```python
from build123d import *

# Parameters (mm, degrees)
SKETCH1_W           = 10
SKETCH1_H           = 10
SKETCH1_W_2         = 8
SKETCH1_H_2         = 8
BOSS_EXTRUDE1_DEPTH = 500
CUT_EXTRUDE1_REACH  = 502.125
SKETCH2_R           = 1.6
CUT_EXTRUDE2_REACH  = 502.125
SKETCH3_R           = 1.6
SKETCH4_R           = 1.6
CUT_EXTRUDE3_DEPTH  = 10
SKETCH5_R           = 3.25
CUT_EXTRUDE4_DEPTH  = 1


with BuildPart() as part:
    # Sketch1 → Boss-Extrude1 (new body)
    with BuildSketch(Plane.XY):
        Rectangle(SKETCH1_W, SKETCH1_H)
        Rectangle(SKETCH1_W_2, SKETCH1_H_2, mode=Mode.SUBTRACT)
    extrude(amount=BOSS_EXTRUDE1_DEPTH)

    # Cut-Extrude1: up to this face of the body (flat: up to its plane)
    cut_extrude1_end = Plane(part.part.faces().sort_by_distance((0, -5, 250))[0])
    # Sketch2 → Cut-Extrude1 (cut, up to the picked face)
    with BuildSketch(Plane(origin=(0, 5, 0), x_dir=(1, 0, 0), z_dir=(0, 1, 0)), mode=Mode.PRIVATE) as cut_extrude1_sk1:
        with Locations(Location((0, -349.5, 0), (0, 0, 270))):
            Circle(SKETCH2_R)
    cut_extrude1_tool1 = split(extrude(cut_extrude1_sk1.sketch, amount=-CUT_EXTRUDE1_REACH, mode=Mode.PRIVATE), bisect_by=cut_extrude1_end, keep=Keep.BOTH, mode=Mode.PRIVATE)
    add(cut_extrude1_tool1.solids().sort_by(Axis((0, 5, 349.5), (0, -1, 0)))[0], mode=Mode.SUBTRACT)

    # Cut-Extrude2: up to this face of the body (flat: up to its plane)
    cut_extrude2_end = Plane(part.part.faces().sort_by_distance((0, -5, 249.839696857))[0])
    # Sketch3 → Cut-Extrude2 (cut, up to the picked face)
    with BuildSketch(Plane(origin=(0, 5, 0), x_dir=(1, 0, 0), z_dir=(0, 1, 0)), mode=Mode.PRIVATE) as cut_extrude2_sk1:
        with Locations(Location((0, -475, 0), (0, 0, 270))):
            Circle(SKETCH3_R)
    cut_extrude2_tool1 = split(extrude(cut_extrude2_sk1.sketch, amount=-CUT_EXTRUDE2_REACH, mode=Mode.PRIVATE), bisect_by=cut_extrude2_end, keep=Keep.BOTH, mode=Mode.PRIVATE)
    # Sketch3 → Cut-Extrude2 (cut, up to the picked face)
    with BuildSketch(Plane(origin=(0, 5, 0), x_dir=(1, 0, 0), z_dir=(0, 1, 0)), mode=Mode.PRIVATE) as cut_extrude2_sk2:
        with Locations(Location((0, -25, 0), (0, 0, 270))):
            Circle(SKETCH3_R)
    cut_extrude2_tool2 = split(extrude(cut_extrude2_sk2.sketch, amount=-CUT_EXTRUDE2_REACH, mode=Mode.PRIVATE), bisect_by=cut_extrude2_end, keep=Keep.BOTH, mode=Mode.PRIVATE)
    add(cut_extrude2_tool1.solids().sort_by(Axis((0, 5, 475), (0, -1, 0)))[0], mode=Mode.SUBTRACT)
    add(cut_extrude2_tool2.solids().sort_by(Axis((0, 5, 25), (0, -1, 0)))[0], mode=Mode.SUBTRACT)

    # Sketch4 → Cut-Extrude3 (cut)
    with BuildSketch(Plane(origin=(5, 0, 0), x_dir=(0, 0, -1), z_dir=(1, 0, 0))):
        with Locations(Location((-70, 0, 0), (0, 0, 90))):
            Circle(SKETCH4_R)
        with Locations(Location((-90, 0, 0), (0, 0, 90))):
            Circle(SKETCH4_R)
        with Locations(Location((-394.5, 0, 0), (0, 0, 90))):
            Circle(SKETCH4_R)
        with Locations(Location((-379.5, 0, 0), (0, 0, 90))):
            Circle(SKETCH4_R)
    extrude(amount=-CUT_EXTRUDE3_DEPTH, mode=Mode.SUBTRACT)

    # Sketch5 → Cut-Extrude4 (cut)
    with BuildSketch(Plane(origin=(0, 5, 0), x_dir=(1, 0, 0), z_dir=(0, 1, 0))):
        with Locations(Location((0, -349.5, 0), (0, 0, 270))):
            Circle(SKETCH5_R)
    extrude(amount=-CUT_EXTRUDE4_DEPTH, mode=Mode.SUBTRACT)


solid = part.part
```
CAD build for the part. Positions are in the model's coordinates, mm. A direction names the side the tool comes from. Coordinates: 2 decimals unless noted, no trailing zeros. Order: outer loops, then holes, each group sorted by start corner. A loop starts at its lowest first (then second) coordinate and runs counter-clockwise, first axis right, second up. Notation, with made-up numbers: M -6,78.25 L 10,78.25 A20 cw 10,84.25 Z; hole C -25,14 d4. An arc over 180 degrees is marked long. Write each question's results on one line, items separated by ' | '. Start each with the question number.
Q1. Drill centre lines: probe 1 along Z at (x, y) = (-4.7, 0); probe 2 along Y at (x, z) = (4.7, 90); probe 3 along X at (y, z) = (0, 340.5). Where is each one in solid material? Low to high. Write a range as from..to.
Q2. Cut at A-A (z = 329). List the corners of the cut face in (x, y).
Q3. Pull direction X, two halves, no side cores. Call faces 3 (the flat face through (-4, 0, 246)), 4 (the flat face through (5, 0, 246)), 5 (the flat face through (-4.5, 0.1, 0)): +X half, -X half, draft (parallel to the pull), parting line (faces both ways), or undercut.
Q4. Which spindle directions (+Z, -Z, +X, -X, +Y, -Y) get a long thin tool onto all of the face, cutting with end or side? Do faces 1 (the flat face through (0, -5, 246)), 2 (the flat face through (0, -4, 246)). Say none if no direction does.
Q5. Flat gauge pin, fed straight in: P1, Ø6, axis at x = -1.5, y = 3, coming from the +Z side. Where does the tip first touch, or does it go through?
Q6. Cut at B-B (y = 0). Count the separate pieces of the cut face and the enclosed holes in it, then the cut area to 3 significant figures.
Found:
1) probe 1: 0..68.4, 71.6..88.4, 91.6..377.9, 381.1..392.9, 396.1..500 | probe 2: -5..-1.6, 1.6..5 | probe 3: -5..-4, 4..5
2) outline: M -5,-5 L 5,-5 L 5,5 L -5,5 Z; hole M -4,-4 L 4,-4 L 4,4 L -4,4 Z
3) face 3: undercut | face 4: +X half | face 5: draft
4) face 1: +Z, -Z, +X, -X, -Y | face 2: +Z, -Z
5) P1: z = 500
6) separate pieces: 10 | enclosed holes: 0 | area: 974 mm²
